```python
from build123d import *

# Parameters (mm, degrees)
F1_DEPTH = 10
F2_R     = 6
F3_DEPTH = 10
F2_R_2   = 8.05
F2_R_3   = 0.9
F4_DEPTH = 5.1
F7_DEPTH = 6.7


with BuildPart() as f1:
    # F0 (on Top) → F1 (new body)
    with BuildSketch(Plane.XY):
        with BuildLine():
            Line((-5, 14.5), (-5, 10.3561575886))
            ThreePointArc((-5, 10.3561575886), (0, 11.5), (5, 10.3561575886))
            Line((5, 10.3561575886), (5, 14.5))
            Line((5, 14.5), (20, 14.5))
            Line((20, 14.5), (20, 19.5))
            Line((20, 19.5), (14.5, 19.5))
            Line((14.5, 19.5), (12.8, 21.2))
            Line((12.8, 21.2), (7.2, 21.2))
            Line((7.2, 21.2), (5.5, 19.5))
            Line((5.5, 19.5), (-5.5, 19.5))
            Line((-5.5, 19.5), (-7.2, 21.2))
            Line((-7.2, 21.2), (-12.8, 21.2))
            Line((-12.8, 21.2), (-14.5, 19.5))
            Line((-14.5, 19.5), (-20, 19.5))
            Line((-20, 19.5), (-20, 14.5))
            Line((-20, 14.5), (-5, 14.5))
        make_face()
        with BuildLine():
            ThreePointArc((-5, 10.3561575886), (-11.2103927672, -2.5645845676), (5.56e-08, -11.5))
            ThreePointArc((5.56e-08, -11.5), (8.1317280033, -8.131727964), (11.5, 0))
            ThreePointArc((11.5, 0), (9.7403798694, 6.1135096303), (5, 10.3561575886))
            ThreePointArc((5, 10.3561575886), (0, 11.5), (-5, 10.3561575886))
        make_face()
    extrude(amount=F1_DEPTH)

    # F2 (on face) → F3 (cut, through all)
    with BuildSketch(Plane.XY.offset(10)):
        Circle(F2_R)
    extrude(amount=-F3_DEPTH, mode=Mode.SUBTRACT)

    # F2 (on face) → F4 (cut)
    with BuildSketch(Plane.XY.offset(10)):
        Circle(F2_R_2)
        Circle(F2_R, mode=Mode.SUBTRACT)
        with Locations((-8.227241336, -4.75)):
            Circle(F2_R_3)
        with Locations((0, 9.5)):
            Circle(F2_R_3)
        with Locations((8.227241336, -4.75)):
            Circle(F2_R_3)
    extrude(amount=-F4_DEPTH, mode=Mode.SUBTRACT)

    # F6 (on offset) → F7 (cut, through all)
    with BuildSketch(Plane(origin=(0, 21.2, 0), x_dir=(-1, 0, 0), z_dir=(0, 1, 0))):
        with BuildLine():
            ThreePointArc((10, 2.45), (11.803122292, 3.196877708), (12.55, 5))
            ThreePointArc((12.55, 5), (11.803122292, 6.803122292), (10, 7.55))
            ThreePointArc((10, 7.55), (7.45, 5), (10, 2.45))
        make_face()
        with BuildLine():
            ThreePointArc((10, 7.55), (11.803122292, 6.803122292), (12.55, 5))
            ThreePointArc((12.55, 5), (11.803122292, 3.196877708), (10, 2.45))
            Line((10, 2.45), (20, 2.45))
            Line((20, 2.45), (20, 7.55))
            Line((20, 7.55), (10, 7.55))
        make_face()
        with BuildLine():
            ThreePointArc((-10, 2.45), (-12.55, 5), (-10, 7.55))
            Line((-10, 7.55), (-20, 7.55))
            Line((-20, 7.55), (-20, 2.45))
            Line((-20, 2.45), (-10, 2.45))
        make_face()
        with BuildLine():
            ThreePointArc((-10, 2.45), (-8.196877708, 3.196877708), (-7.45, 5))
            ThreePointArc((-7.45, 5), (-8.196877708, 6.803122292), (-10, 7.55))
            ThreePointArc((-10, 7.55), (-12.55, 5), (-10, 2.45))
        make_face()
    extrude(amount=-F7_DEPTH, mode=Mode.SUBTRACT)


solid = f1.part
```
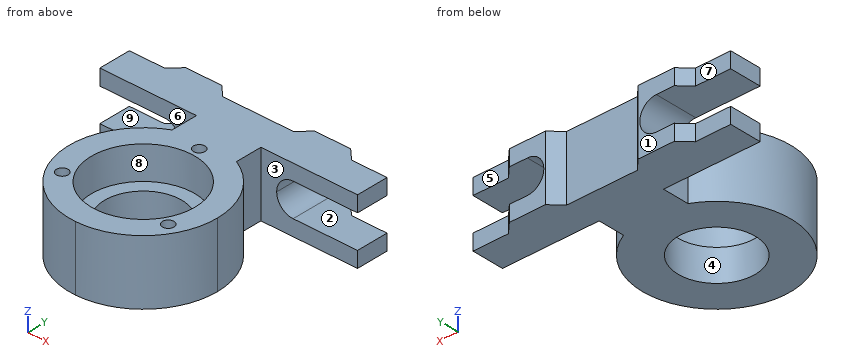
The model under review builds one solid part; all positions refer to its coordinate system, in mm. Face numbers are marked on the shaded views. A direction names the side the tool comes from. Round coordinates to 2 decimals unless told otherwise and drop trailing zeros. Loops run counter-clockwise (first coordinate to the right, second up) from the corner with the lowest first, then second, coordinate; pieces in that order, holes last.
Item 1: For line 1 (X direction, y = -5, z = 8.25); line 2 (X direction, y = -4, z = 6.25); line 3 (X direction, y = 11, z = 7), list the stretches that pass through material, from the lowest coordinate up.
Determined:
line 1: x = -10.36 to -9.09, -7.36 to -6.31, 6.31 to 7.36, 9.09 to 10.36
line 2: x = -10.78 to -8.72, -7.73 to -6.99, 6.99 to 7.73, 8.72 to 10.78
line 3: x = -5 to 5
Item 2: For the marked faces 5, 6, 7, 8 and 9, list the 3-axis set-ups (+Z, -Z, +X, -X, +Y, -Y) from which the entire face can be reached by the end or side of a thin tool; tool diameter is ignored.
Determined:
face 5: +Z, -Z, +X, +Y
face 6: +Z, -Z, -X
face 7: +Z, -Z, -X, +Y
face 8: +Z
face 9: -X, +Y
Item 3: Mouldability with a two-part tool opening along Y and no side actions: class the marked faces 1, 2, 3 and 4 as released by +Y, released by -Y, zero draft, split by the parting line, or undercut.
Determined:
face 1: released by +Y
face 2: zero draft
face 3: undercut
face 4: undercut
Item 4: Take a section at A-A (y = -2). Write out the cut boundary in (x, z), then the cut area to 3 significant figures.
Determined:
outline: (-11.32, 0) - (-5.66, 0) - (-5.66, 4.9) - (-7.8, 4.9) - (-7.8, 10) - (-11.32, 10) - close; (5.66, 0) - (11.32, 0) - (11.32, 10) - (7.8, 10) - (7.8, 4.9) - (5.66, 4.9) - close
area: 91.5 mm2
Item 5: Clearance check with flat-ended pins moving along their axes: pin 1 Ø0.7 at (x, z) = (-16.5, 9) entering from +Y; pin 2 Ø14.5 at (x, y) = (0, 0) entering from +Z; pin 3 Ø4 at (y, z) = (-7.5, 8) entering from -X; pin 4 Ø4 at (x, z) = (11, 3.5) entering from +Y. State where each tip first meets the part, or that it passes through.
Determined:
pin 1: stops at y = 19.5
pin 2: stops at z = 4.9
pin 3: stops at x = -10.1
pin 4: stops at y = 21.2
Item 6: Take a section at C-C (z = 2). Write out the cut boundary in (x, y).
Determined:
outline: (-20, 14.5) - (-5, 14.5) - (-5, 10.36) arc R11.5 ccw (long way) to (5, 10.36) - (5, 14.5) - (20, 14.5) - (20, 19.5) - (14.5, 19.5) - (12.8, 21.2) - (7.2, 21.2) - (5.5, 19.5) - (-5.5, 19.5) - (-7.2, 21.2) - (-12.8, 21.2) - (-14.5, 19.5) - (-20, 19.5) - close; hole circle Ø12 at (0, 0)
Item 7: Take a section at B-B (z = 8.5). Write out the cut boundary in (x, y), then the cut area to 3 significant figures.
Determined:
outline: (-20, 14.5) - (-5, 14.5) - (-5, 10.36) arc R11.5 ccw (long way) to (5, 10.36) - (5, 14.5) - (20, 14.5) - (20, 19.5) - (14.5, 19.5) - (12.8, 21.2) - (7.2, 21.2) - (5.5, 19.5) - (-5.5, 19.5) - (-7.2, 21.2) - (-12.8, 21.2) - (-14.5, 19.5) - (-20, 19.5) - close; hole circle Ø1.8 at (-8.23, -4.75); hole circle Ø16.1 at (0, 0); hole circle Ø1.8 at (0, 9.5); hole circle Ø1.8 at (8.23, -4.75)
area: 463 mm2
Item 8: Take a section at D-D (y = 17). Write out the cut boundary in (x, z).
Determined:
outline: (-20, 0) - (20, 0) - (20, 2.45) - (10, 2.45) arc R2.55 cw to (10, 7.55) - (20, 7.55) - (20, 10) - (-20, 10) - (-20, 7.55) - (-10, 7.55) arc R2.55 cw to (-10, 2.45) - (-20, 2.45) - close
